Geometry: final body of the model. Coordinates: model frame, mm. A direction names the side the tool comes from. Coordinates: 2 decimals unless noted, no trailing zeros. Order: outer loops, then holes, each group sorted by start corner. A loop starts at its lowest first (then second) coordinate and runs counter-clockwise, first axis right, second up. Notation, with made-up numbers: (-5, -24) -> (12, -24) arc R23 cw to (12, 8) -> close; hole circle Ø1 at (-36, 79.25). An arc over 180 degrees is marked (long way). Answer in a Markdown table with one row per item. Add a question column.
1) Contact query for flat-ended pins moving along their axis: P1, Ø2.5, axis at x = -49, z = 249, coming from the +Y side; P2, Ø12, axis at x = -33, z = 223, coming from the +Y side. Output: stop coordinate, or through.
2) Section query B-B on y = -5. Count the separate pieces of the cut face and the enclosed holes in it, then the cut area to 3 significant figures.
3) Pull-direction query (X, two-part tool) for faces 4 (the face through (-60.65, -4.93, 160.31)), 5 (the face through (-16, -1.5, 221)), 6 (the face through (-33, -5, 0)); classes: +X half, -X half, draft (parallel to the pull), parting line (faces both ways), or undercut.
4) Section query C-C on x = -11. Return the cut outline in (y, z), then the cut area to 3 significant figures.
5) Set-up query: faces 1 (the face through (-27.6, -0.74, 244.83)), 2 (the face through (-27, -5, 300)), 3 (the face through (-60, -5, 233)). Return all of +Z, -Z, +X, -X, +Y, -Y with unobstructed straight access to the full face (end or side cutting, diameter ignored); none if empty.
6) Section query A-A on x = -25. Return the cut outline in (y, z), then the cut area to 3 significant figures.
7) Ray query, line 1 (Z direction, x = -59, y = -2.5); line 2 (X direction, y = -7.5, z = 249); line 3 (Z direction, x = -1, y = -7). Return the intervals inside material, ascending. Write a range as from..to.
```python
from build123d import *

# Parameters (mm, degrees)
F0_R     = 2.5
F0_R_2   = 2
F0_R_3   = 20
F0_R_4   = 9
F1_DEPTH = 10
F2_R     = 2
F3_DEPTH = 15
F4_DEPTH = 1.5


with BuildPart() as f1:
    # F0 (on Front) → F1 (new body)
    with BuildSketch(Plane.XZ):
        with BuildLine():
            Line((-70, 0), (0, 0))
            Line((0, 0), (0, 199.267949))
            ThreePointArc((0, 199.267949), (-3, 201), (0, 202.732051))
            Line((0, 202.732051), (0, 247.267949))
            ThreePointArc((0, 247.267949), (-3, 249), (0, 250.732051))
            Line((0, 250.732051), (0, 300))
            Line((0, 300), (-60, 300))
            Line((-60, 300), (-60, 163.85171))
            ThreePointArc((-60, 163.85171), (-60.668282, 160.257403), (-62.583808, 157.143498))
            Line((-62.583808, 157.143498), (-67.416192, 151.801108))
            ThreePointArc((-67.416192, 151.801108), (-69.331718, 148.687203), (-70, 145.092897))
            Line((-70, 145.092897), (-70, 0))
        make_face()
        with Locations((-59, 6)):
            Circle(F0_R, mode=Mode.SUBTRACT)
        with Locations((-59, 36)):
            Circle(F0_R, mode=Mode.SUBTRACT)
        with Locations((-11, 6)):
            Circle(F0_R, mode=Mode.SUBTRACT)
        with Locations((-11, 36)):
            Circle(F0_R, mode=Mode.SUBTRACT)
        with Locations((-49, 201)):
            Circle(F0_R_2, mode=Mode.SUBTRACT)
        with Locations((-49, 249)):
            Circle(F0_R_2, mode=Mode.SUBTRACT)
        with Locations((-4.837179, 155)):
            Circle(F0_R_2, mode=Mode.SUBTRACT)
        with Locations((-5.474639, 185)):
            Circle(F0_R_2, mode=Mode.SUBTRACT)
        with Locations((-25, 225)):
            Circle(F0_R_3, mode=Mode.SUBTRACT)
        with Locations((-4.837179, 265)):
            Circle(F0_R_2, mode=Mode.SUBTRACT)
        with Locations((-4.837179, 295)):
            Circle(F0_R_2, mode=Mode.SUBTRACT)
        with Locations((-25, 225)):
            Circle(F0_R_3)
        with Locations((-25, 225)):
            Circle(F0_R_4, mode=Mode.SUBTRACT)
        with BuildLine():
            Line((0, 199.267949), (0, 0))
            Line((0, 0), (5, 0))
            Line((5, 0), (5, 300))
            Line((5, 300), (0, 300))
            Line((0, 300), (0, 250.732051))
            ThreePointArc((0, 250.732051), (0.732051, 250), (1, 249))
            ThreePointArc((1, 249), (0.732051, 248), (0, 247.267949))
            Line((0, 247.267949), (0, 202.732051))
            ThreePointArc((0, 202.732051), (0.732051, 202), (1, 201))
            ThreePointArc((1, 201), (0.732051, 200), (0, 199.267949))
        make_face()
    extrude(amount=F1_DEPTH)

    # F2 (on face) → F3 (cut)
    with BuildSketch(Plane.XY.offset(300)):
        with Locations((-41, -5)):
            Circle(F2_R)
    extrude(amount=-F3_DEPTH, mode=Mode.SUBTRACT)

    # F0 (on Front) → F4 (cut)
    with BuildSketch(Plane.XZ):
        with Locations((-25, 225)):
            Circle(F0_R_3)
        with Locations((-25, 225)):
            Circle(F0_R_4, mode=Mode.SUBTRACT)
    extrude(amount=F4_DEPTH, mode=Mode.SUBTRACT)


solid = f1.part
```
Result:
| question | item | result |
|---|---|---|
| 1 | P1 | through |
| 1 | P2 | y = -1.5 |
| 2 | separate pieces | 1 |
| 2 | enclosed holes | 13 |
| 2 | area | 20,600 mm2 |
| 3 | face 4 | -X half |
| 3 | face 5 | undercut |
| 3 | face 6 | draft |
| 4 | outline | (-10, 0) -> (0, 0) -> (0, 3.5) -> (-10, 3.5) -> close; (-10, 8.5) -> (0, 8.5) -> (0, 33.5) -> (-10, 33.5) -> close; (-10, 38.5) -> (0, 38.5) -> (0, 210.72) -> (-1.5, 210.72) -> (-1.5, 239.28) -> (0, 239.28) -> (0, 300) -> (-10, 300) -> close |
| 4 | area | 2,860 mm2 |
| 5 | face 1 | +Y |
| 5 | face 2 | +Z, +X, -X, +Y, -Y |
| 5 | face 3 | +Z, -X, +Y, -Y |
| 6 | outline | (-10, 0) -> (0, 0) -> (0, 205) -> (-1.5, 205) -> (-1.5, 216) -> (-10, 216) -> close; (-10, 234) -> (-1.5, 234) -> (-1.5, 245) -> (0, 245) -> (0, 300) -> (-10, 300) -> close |
| 6 | area | 2,790 mm2 |
| 7 | line 1 | 0..3.5, 8.5..33.5, 38.5..300 |
| 7 | line 2 | -60..-51, -47..-3, 1..5 |
| 7 | line 3 | 0..199, 203..247, 251..300 |
